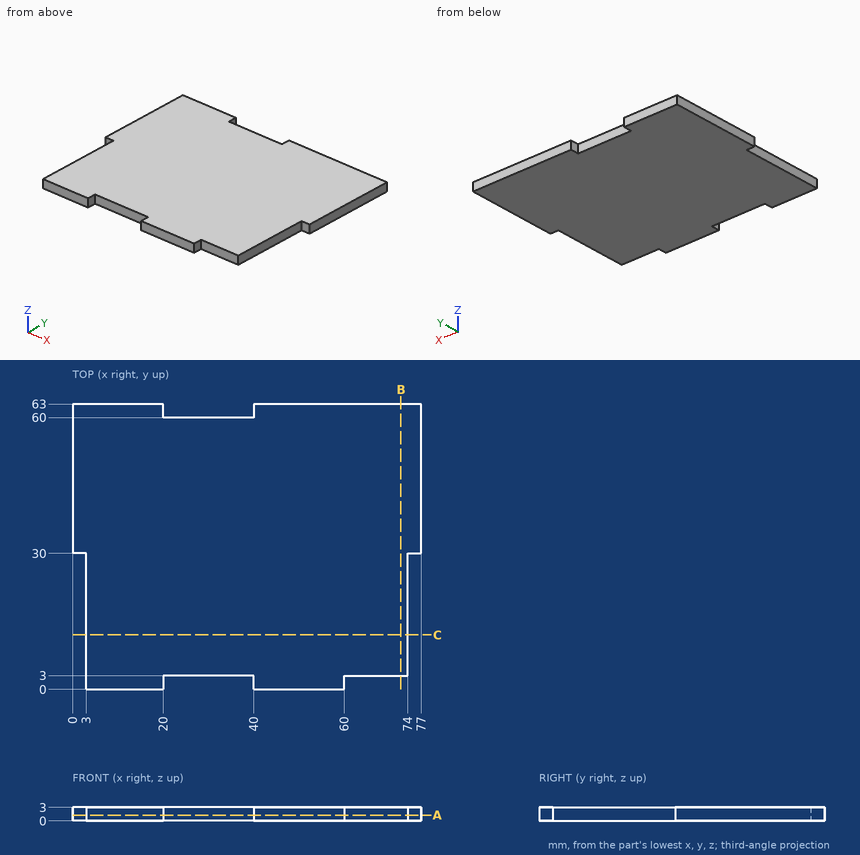
Job drawing, mm, ordinate dimensions from the low corner. One solid piece. Round coordinates to 2 decimals unless told otherwise and drop trailing zeros. Write each loop counter-clockwise with the first axis right and the second up, starting at its lowest first coordinate (ties: lowest second). Pieces come first, ordered by that corner, then holes.
1) Drill centre lines: probe 1 along X at (y, z) = (12, 1.85); probe 2 along Y at (x, z) = (28.5, 1.75); probe 3 along Y at (x, z) = (66, 0.35). Where is each one in solid material? Low to high.
2) Band-saw the part on A-A, the plane z = 1.25. List the corners of the cut face in (x, y), and give its area (3 significant figures).
3) Band-saw the part on C-C, the plane y = 12. List the corners of the cut face in (x, z), and give its area (3 significant figures).
4) Band-saw the part on B-B, the plane x = 72.5. List the corners of the cut face in (y, z).
5) Pin check, flat tips, straight feed: pin 1 (0.9 mm diameter, centred on y = 2, z = 1, fed in from -X); pin 2 (0.9 mm diameter, centred on y = 1, z = 2, fed in from +X); pin 3 (1.5 mm diameter, centred on y = 10, z = 1.5, fed in from +X). Stop position of each tip, or through.
Ans:
1. probe 1: x = 3 to 74
1. probe 2: y = 3 to 60
1. probe 3: y = 3 to 63
2. outline: (0, 30) - (3, 30) - (3, 0) - (20, 0) - (20, 3) - (40, 3) - (40, 0) - (60, 0) - (60, 3) - (74, 3) - (74, 30) - (77, 30) - (77, 63) - (40, 63) - (40, 60) - (20, 60) - (20, 63) - (0, 63) - close
2. area: 4,510 mm2
3. outline: (3, 0) - (74, 0) - (74, 3) - (3, 3) - close
3. area: 213 mm2
4. outline: (3, 0) - (63, 0) - (63, 3) - (3, 3) - close
5. pin 1: stops at x = 3
5. pin 2: stops at x = 60
5. pin 3: stops at x = 74
